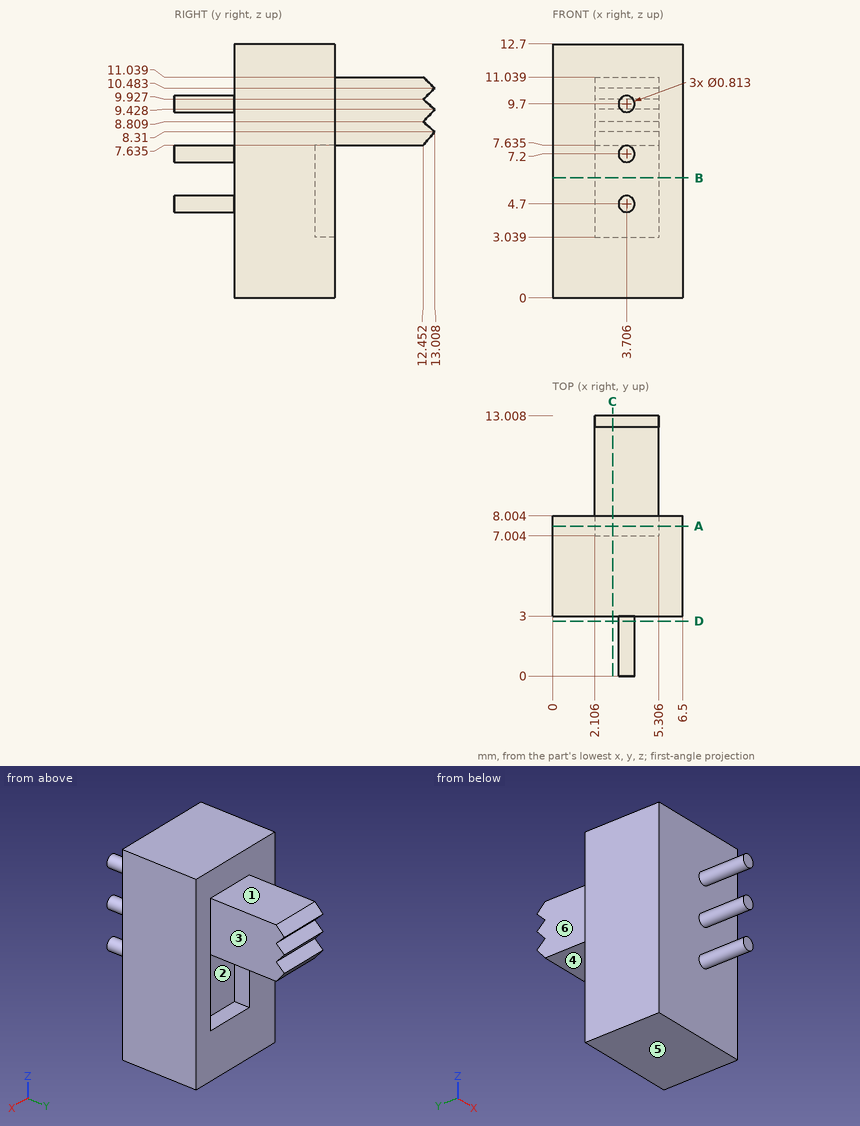
Could you check a few things on this drawing? It's one solid part, dimensions in mm from its lowest x, y, z. A direction names the side the tool comes from. Round coordinates to 2 decimals unless told otherwise and drop trailing zeros. Loops run counter-clockwise (first coordinate to the right, second up) from the corner with the lowest first, then second, coordinate; pieces in that order, holes last. Notation, with made-up numbers: M 72.25,49.25 L 125.25,49.25 A18 ccw 125.25,58.25 Z; hole C 85.5,0 d11. An arc over 180 degrees is marked long. Write item = value, one per line. Start each with the question number.
(1) Suppose I cut it at D-D on y = 2.75. Write out the boundary of the cut face in (x, z).
(2) Suppose I cut it at B-B on z = 6. Write out the boundary of the cut face in (x, y) (1 decimal), plus the area to 3 significant figures.
(3) I'm going to push flat-ended pins straight in: P1, Ø2.5, axis at y = 10.5, z = 10, coming from the +X side; P2, Ø3.5, axis at y = 10.5, z = 9, coming from the -X side; P3, Ø3, axis at x = 1.5, z = 4, coming from the +Y side. Where does each tip first touch, or does it pass through?
(4) Which directions (+Z, -Z, +X, -X, +Y, -Y) give clear straight access to the entire face, cutting with the end or side of a thin tool? Please do the marked faces 1, 2 and 3.
(5) Suppose I cut it at C-C on x = 3. Write out the boundary of the cut face in (y, z) (1 decimal).
(6) Suppose I cut it at A-A on y = 7.5. Write out the boundary of the cut face in (x, z) (1 decimal).
(7) If we mould it in two halves opening along X, with no side actions, what happens to the marked faces 4, 5 and 6? For each: released by +X, released by -X, zero draft, split by the parting line, or undercut.
(8) I need wall thicknesses on line 1 along X through (y, z) = (10, 9) (1 decimal); line 2 along Z through (x, y) = (4, 2.5); line 3 along Y through (x, z) = (6, 0.5). Which ranges of each line are inside material? Lowest first, please.
Answer block:
q1.outline = C 3.71,4.7 d0.81; C 3.71,7.2 d0.81; C 3.71,9.7 d0.81
q2.outline = M 0,3 L 6.5,3 L 6.5,8 L 5.3,8 L 5.3,7 L 2.1,7 L 2.1,8 L 0,8 Z
q2.area = 29.3 mm²
q3.P1 = 5.31
q3.P2 = 2.11
q3.P3 = 8
q4.face_1 = +Z, +X, -X, +Y
q4.face_2 = +Y
q4.face_3 = +Z, -Z, +X, +Y
q5.outline = M 3,0 L 8,0 L 8,3 L 7,3 L 7,7.6 L 12.5,7.6 L 13,8.3 L 12.5,8.8 L 13,9.4 L 12.5,9.9 L 13,10.5 L 12.5,11 L 8,11 L 8,12.7 L 3,12.7 Z
q6.outline = M 0,0 L 6.5,0 L 6.5,12.7 L 0,12.7 Z; hole M 2.1,3 L 5.3,3 L 5.3,7.6 L 2.1,7.6 Z
q7.face_4 = undercut
q7.face_5 = zero draft
q7.face_6 = released by -X
q8.line_1 = 2.1 to 5.3
q8.line_2 = 4.42 to 4.98, 6.92 to 7.48, 9.42 to 9.98
q8.line_3 = 3 to 8
